from build123d import *

# Parameters (mm, degrees)
SKETCH1_R           = 6
SKETCH1_R_2         = 5.2
BOSS_EXTRUDE1_DEPTH = 25
SKETCH2_R           = 6
SKETCH2_R_2         = 5
BOSS_EXTRUDE2_DEPTH = 10


with BuildPart() as part:
    # Sketch1 → Boss-Extrude1 (new body)
    with BuildSketch(Plane(origin=(0, 0, 0), x_dir=(1, 0, 0), z_dir=(0, 1, 0))):
        Circle(SKETCH1_R)
        Circle(SKETCH1_R_2, mode=Mode.SUBTRACT)
    extrude(amount=BOSS_EXTRUDE1_DEPTH)

    # Sketch2 → Boss-Extrude2 (add)
    with BuildSketch(Plane(origin=(0, 25, 0), x_dir=(1, 0, 0), z_dir=(0, 1, 0))):
        Circle(SKETCH2_R)
        Circle(SKETCH2_R_2, mode=Mode.SUBTRACT)
    extrude(amount=BOSS_EXTRUDE2_DEPTH)

    # Sketch3 → Revolve2 (revolve)
    with BuildSketch(Plane(origin=(0, 0, 0), x_dir=(0, 0, -1), z_dir=(1, 0, 0))):
        with BuildLine():
            Line((-6, 35), (-2, 35))
            Line((-2, 35), (-1.559699238, 35))
            Line((-1.559699238, 35), (-2, 35.440300762))
            ThreePointArc((-2, 35.440300762), (-4.012879655, 37.197699204), (-4.7625, 39.7625))
            Line((-4.7625, 39.7625), (-5.5125, 39.7625))
            Line((-5.5125, 39.7625), (-6, 35))
        make_face()
    revolve(axis=Axis((0, 33.973403882, 0), (0, -1, 0)))


solid = part.part
The listing builds one solid part. Answer for the finished solid, in the listing's coordinates (mm). A direction names the side the tool comes from. Give positions to 0.01 mm unless a question says otherwise; leave off trailing zeros. Loops run counter-clockwise (first coordinate to the right, second up) from the corner with the lowest first, then second, coordinate; pieces in that order, holes last. Notation, with made-up numbers: (40.5, -11) - (96.5, -11) arc R18 cw to (96.5, 5) - close; hole circle Ø7 at (35, 21). An arc over 180 degrees is marked (long way). Write each question's results on one line, items separated by ' | '.
1. For a pull along Z with two mould halves and no side action, classify faces 1 (the face through (-6, 17, 0)), 2 (the face through (-1.08, 29.93, 4.88)), 3 (the face through (-2, 0, -5)) as +Z half, -Z half, draft (parallel to the pull), parting line (faces both ways), or undercut.
Resolved:
face 1: parting line | face 2: undercut | face 3: draft
2. Which of the six approach directions +Z, -Z, +X, -X, +Y, -Y give full straight-line access (tool end or side, diameter ignored) to faces 4 (the face through (0, 39.762, 5)), 5 (the face through (-0.677, 12.325, -5.156))?
Resolved:
face 4: +Z, -Z, +X, -X, +Y | face 5: -Y
3. Find section A-A, the plane y = 28.5. Write down the section's boundary in (x, z), then the cut area to 3 significant figures.
Resolved:
outline: circle Ø12 at (0, 0); hole circle Ø10 at (0, 0) | area: 34.6 mm^2
4. Consider probe 1 along Z at (x, y) = (0, 28.25); probe 2 along Z at (x, y) = (0, 19.25). Determine where each line is inside the solid, lowest interval first. Write a range as from..to.
Resolved:
probe 1: z = -6..-5, 5..6 | probe 2: z = -6..-5.2, 5.2..6
5. Flat-ended cylindrical pins translate along their axes: P1, Ø2, axis at y = 29.5, z = 3, coming from the -X side; P2, Ø5, axis at x = -1, z = 2, coming from the -Y side; P3, Ø1.5, axis at x = 4.5, y = 27, coming from the -Z side; P4, Ø1.5, axis at x = 0.5, y = 34.5, coming from the +Z side. Find the tip coordinate at first contact, or state that the pin passes through.
Resolved:
P1: stops at x = -5.66 | P2: stops at y = 35 | P3: stops at z = -4.68 | P4: stops at z = 6
6. Find section D-D, the plane y = 14. Write down the section's boundary in (x, z).
Resolved:
outline: circle Ø12 at (0, 0); hole circle Ø10.4 at (0, 0)
